```python
from build123d import *

# Parameters (mm, degrees)
BOSS_EXTRUDE1_DEPTH     = 40
SKETCH2_W               = 13.73333333
SKETCH2_H               = 6
CUT_EXTRUDE1_DEPTH      = 58.827329179
SKETCH3_W               = 40
SKETCH3_H               = 11.8
BOSS_EXTRUDE2_DEPTH     = 4
BOSS_EXTRUDE3_DEPTH     = 13.73333333
SKETCH10_R              = 1.47
BOSS_EXTRUDE7_DEPTH     = 5.5
SKETCH13_W              = 40
SKETCH13_H              = 44
BOSS_EXTRUDE8_DEPTH     = 19.5
CHAMFER2_START          = -20
CHAMFER2_DEPTH          = 5.5
EXTRUDE_THIN1_START     = -3
SKETCH14_R              = 9.05
SKETCH14_R_2            = 6.05
EXTRUDE_THIN1_DEPTH     = 8
BOSS_EXTRUDE9_START     = 3
BOSS_EXTRUDE9_DEPTH     = 3
FILLET1_START           = -31.5
FILLET1_DEPTH           = 11
SKETCH16_W              = 30
SKETCH16_H              = 18.101031733
CUT_EXTRUDE4_DEPTH      = 37.5
CHAMFER1_SIZE           = 14
CHAMFER1_SIZE2          = 18.1
SKETCH17_R              = 1.45
CUT_EXTRUDE5_DEPTH      = 35
SKETCH18_R              = 6.05
CUT_EXTRUDE6_DEPTH      = 16
FILLET2_R               = 0.6
CUT_EXTRUDE7_DEPTH      = 58.690987254
CUT_EXTRUDE7_DEPTH_BACK = 10


with BuildPart() as part:
    # Sketch1 → Boss-Extrude1 (new body)
    with BuildSketch(Plane.XY):
        Polygon((-20, -0.2), (-20, -12), (20, -12), (20, -0.2), (14.253501692, -0.2), (14.253501692, -1.22065898), (16.532842712, -3.5), (13.832842712, -6.2), (6.167157288, -6.2), (3.467157288, -3.5), (5.746498308, -1.22065898), (5.746498308, -0.2), (-5.746498308, -0.2), (-5.746498308, -1.22065898), (-3.467157288, -3.5), (-6.167157288, -6.2), (-13.832842712, -6.2), (-16.532842712, -3.5), (-14.253501692, -1.22065898), (-14.253501692, -0.2), align=None)
    extrude(amount=-BOSS_EXTRUDE1_DEPTH)

    # Sketch2 → Cut-Extrude1 (cut, through all)
    with BuildSketch(Plane.ZY.offset(20)):
        with Locations((-20, -3.2)):
            Rectangle(SKETCH2_W, SKETCH2_H)
    extrude(amount=-CUT_EXTRUDE1_DEPTH, mode=Mode.SUBTRACT)

    # Sketch3 → Boss-Extrude2 (add)
    with BuildSketch(Plane.XY):
        with Locations((0, -6.1)):
            Rectangle(SKETCH3_W, SKETCH3_H)
    extrude(amount=BOSS_EXTRUDE2_DEPTH)

    # Sketch4 → Boss-Extrude3 (add)
    with BuildSketch(Plane.XY.offset(-26.866666665)):
        Polygon((-20, -0.2), (-20, -6.2), (-13.832842712, -6.2), (-16.532842712, -3.5), align=None)
        Polygon((-6.167157288, -6.2), (6.167157288, -6.2), (3.467157288, -3.5), (0, -0.2), (-3.467157288, -3.5), align=None)
        Polygon((13.832842712, -6.2), (20, -6.2), (20, -0.2), (16.532842712, -3.5), align=None)
    extrude(amount=BOSS_EXTRUDE3_DEPTH)

    # Sketch10 → Boss-Extrude7 (add)
    with BuildSketch(Plane.ZY.offset(20)):
        with BuildLine():
            Line((-40, -12.8), (-42.5, -12.8))
            ThreePointArc((-42.5, -12.8), (-46.5, -8.8), (-42.5, -4.8))
            Line((-42.5, -4.8), (-40, -4.8))
            ThreePointArc((-40, -4.8), (-36, -8.8), (-40, -12.8))
        make_face()
        with Locations((-42.5, -8.8)):
            Circle(SKETCH10_R, mode=Mode.SUBTRACT)
    boss_extrude7 = extrude(amount=-BOSS_EXTRUDE7_DEPTH)

    # Sketch13 → Boss-Extrude8 (add)
    with BuildSketch(Plane.XZ.offset(12)):
        with Locations((0, -18)):
            Rectangle(SKETCH13_W, SKETCH13_H)
    extrude(amount=BOSS_EXTRUDE8_DEPTH)

    # Chamfer2: read off the stored shape, not the designer's step
    # Chamfer2 outline → Chamfer2 (add)
    with BuildSketch(Plane.YZ.offset(CHAMFER2_START)):
        with BuildLine():
            Line((-20.621590418, -40), (-12.177597262, -44.642857143))
            ThreePointArc((-12.177597262, -44.642857143), (-12.641249084, -43.615708508), (-12.8, -42.5))
            Line((-12.8, -42.5), (-12.8, -40))
            Line((-12.8, -40), (-20.621590418, -40))
        make_face()
    chamfer2 = extrude(amount=CHAMFER2_DEPTH)

    # Mirror1: Boss-Extrude7, Chamfer2 across plane
    add(boss_extrude7.mirror(Plane(origin=(0, 0, 0), x_dir=(0, 0, 1), z_dir=(1, 0, 0))))
    add(chamfer2.mirror(Plane(origin=(0, 0, 0), x_dir=(0, 0, 1), z_dir=(1, 0, 0))))

    # Sketch14 → Extrude-Thin1 (add)
    with BuildSketch(Plane.XZ.offset(31.5).offset(EXTRUDE_THIN1_START)):
        with Locations((-0.2, -42.5)):
            Circle(SKETCH14_R)
        with Locations((-0.2, -42.5)):
            Circle(SKETCH14_R_2, mode=Mode.SUBTRACT)
    extrude(amount=-EXTRUDE_THIN1_DEPTH)

    # Sketch15 → Boss-Extrude9 (add)
    with BuildSketch(Plane.XZ.offset(28.5).offset(BOSS_EXTRUDE9_START)):
        with BuildLine():
            Line((8.497844561, -40), (-8.897844561, -40))
            ThreePointArc((-8.897844561, -40), (-0.2, -51.55), (8.497844561, -40))
        make_face()
    extrude(amount=-BOSS_EXTRUDE9_DEPTH)

    # Fillet1: read off the stored shape, not the designer's step
    # Fillet1 outline → Fillet1 (add)
    with BuildSketch(Plane(origin=(0, 0, 0), x_dir=(1, 0, 0), z_dir=(0, 1, 0)).offset(FILLET1_START)):
        with BuildLine():
            ThreePointArc((20, 40), (12.845609752, 42.00741501), (7.532507128, 47.202215809))
            ThreePointArc((7.532507128, 47.202215809), (8.769787751, 43.7022511), (8.497844561, 40))
            Line((8.497844561, 40), (20, 40))
        make_face()
        with BuildLine():
            ThreePointArc((-8.897844561, 40), (-9.170229006, 43.698954374), (-7.935961427, 47.196530719))
            ThreePointArc((-7.935961427, 47.196530719), (-13.07347783, 42.098748758), (-20, 40))
            Line((-20, 40), (-8.897844561, 40))
        make_face()
    extrude(amount=FILLET1_DEPTH)

    # Sketch16 → Cut-Extrude4 (cut)
    with BuildSketch(Plane.XY.offset(4)):
        with Locations((0, -22.449484134)):
            Rectangle(SKETCH16_W, SKETCH16_H)
    extrude(amount=-CUT_EXTRUDE4_DEPTH, mode=Mode.SUBTRACT)

    # Chamfer1
    chamfer1_edges = [part.edges().sort_by_distance(p)[0] for p in [
        (0, -13.398968267, -33.5),
    ]]
    chamfer1_side = [part.faces().sort_by_distance(p)[0] for p in [
        (0, -13.398968267, -14.75),
    ]]
    chamfer(chamfer1_edges, length=CHAMFER1_SIZE, length2=CHAMFER1_SIZE2, reference=chamfer1_side[0])

    # Sketch17 → Cut-Extrude5 (cut)
    with BuildSketch(Plane.ZY.offset(20)):
        with Locations((-4, -26.5)):
            Circle(SKETCH17_R)
        with Locations((-25, -26.5)):
            Circle(SKETCH17_R)
    cut_extrude5 = extrude(amount=-CUT_EXTRUDE5_DEPTH, mode=Mode.SUBTRACT)

    # Mirror3: Cut-Extrude5 across plane
    add(cut_extrude5.mirror(Plane(origin=(0, 0, 0), x_dir=(0, 0, 1), z_dir=(1, 0, 0))), mode=Mode.SUBTRACT)

    # Sketch18 → Cut-Extrude6 (cut)
    with BuildSketch(Plane(origin=(0, -28.5, 0), x_dir=(1, 0, 0), z_dir=(0, 1, 0))):
        with Locations(Location((-0.2, 42.5, 0), (0, 0, 90))):
            Circle(SKETCH18_R)
    extrude(amount=CUT_EXTRUDE6_DEPTH, mode=Mode.SUBTRACT)

    # Fillet2
    fillet2_edges = [part.edges().sort_by_distance(p)[0] for p in [
        (16.695998577, -20.5, -40.066855447),
        (-16.826940077, -20.5, -40.066855447),
    ]]
    fillet(fillet2_edges, radius=FILLET2_R)

    # Sketch19 → Cut-Extrude7 (cut, two sides: drawn at the far end of the back side and taken through both)
    with BuildSketch(Plane(origin=(0, 0, -40), x_dir=(-1, 0, 0), z_dir=(0, 0, -1)).offset(-CUT_EXTRUDE7_DEPTH_BACK)):
        Polygon((16.532842712, -3.5), (15.232842712, -4.8), (14.5, -5.532842712), (13.832842712, -6.2), (10, -6.2), (10, -3.5), align=None)
        Polygon((-13.832842712, -6.2), (-14.5, -5.532842712), (-15.232842712, -4.8), (-16.532842712, -3.5), (-10, -3.5), (-10, -6.2), align=None)
    extrude(amount=CUT_EXTRUDE7_DEPTH + CUT_EXTRUDE7_DEPTH_BACK, mode=Mode.SUBTRACT)


solid = part.part
```
Geometry: final body of the model. Coordinates: model frame, mm. A direction names the side the tool comes from. Round coordinates to 2 decimals unless told otherwise and drop trailing zeros. Order: outer loops, then holes, each group sorted by start corner. A loop starts at its lowest first (then second) coordinate and runs counter-clockwise, first axis right, second up. Notation, with made-up numbers: (-3.75, 78) - (24.25, 78) arc R15 ccw to (24.25, 99) - close; hole circle Ø4 at (7.5, 41). An arc over 180 degrees is marked (long way). Write item = value, one per line. Start each with the question number.
Q1. Cut plane C-C on z = -10.5. Return the cut outline in (x, y), and give its area (3 significant figures).
Q2. Pin query (flat end, axial travel): pin 1 (3.5 mm diameter, centred on x = -16, y = -2, fed in from -Z); pin 2 (1 mm diameter, centred on x = -9, y = -23.5, fed in from +Z); pin 3 (3.5 mm diameter, centred on y = -8.8, z = -42.5, fed in from -X); pin 4 (1 mm diameter, centred on y = -22.5, z = -45.5, fed in from -X). Return the tip coordinate at first contact, or that it passes through.
Q3. Cut plane B-B on z = -4. Give the number of separate pieces and of enclosed holes in the cut face, and give its area (3 significant figures).
Q4. Pull-direction query (Y, two-part tool) for faces 5 (the flat face through (0, -9, 4)), 6 (the cylindrical face through (17.29, -7.75, -46.36)), 7 (the flat face through (4.591, -2.376, -33.341)), 8 (the flat face through (-17, -0.2, -33)); classes: +Y half, -Y half, draft (parallel to the pull), parting line (faces both ways), or undercut.
Q5. Cut plane D-D on y = -26.5. Return the cut outline in (x, z), and give its area (3 significant figures).
Q6. Cut plane A-A on y = -8.8. Return the cut outline in (x, z), and give its area (3 significant figures).
Q7. Ray query, line 1 (X direction, y = -14, z = -8.5); line 2 (Y direction, x = 18, z = -4); line 3 (X direction, y = -12, z = -43.5). Return the intervals inside material, ascending. Write a range as from..to.
Q8. Access query for faces 1 (the cylindrical face through (12.937, -25.639, -41.955)), 2 (the flat face through (-18, -2, -40)), 3 (the flat face through (-0.21, -22.58, -26.6)), 4 (the flat face through (4.591, -2.376, -6.475)). Directions: +Z, -Z, +X, -X, +Y, -Y. A direction counts if a zero-diameter tool reaches every point of the face in a straight line with its end or side. Return the directions, or none.
Outcome:
q1.outline = (-20, -31.5) - (-15, -31.5) - (-15, -13.4) - (15, -13.4) - (15, -31.5) - (20, -31.5) - (20, -0.2) - (14.25, -0.2) - (14.25, -1.22) - (16.53, -3.5) - (13.83, -6.2) - (6.17, -6.2) - (3.47, -3.5) - (5.75, -1.22) - (5.75, -0.2) - (-5.75, -0.2) - (-5.75, -1.22) - (-3.47, -3.5) - (-6.17, -6.2) - (-13.83, -6.2) - (-16.53, -3.5) - (-14.25, -1.22) - (-14.25, -0.2) - (-20, -0.2) - close
q1.area = 586 mm^2
q2.pin_1 = -40
q2.pin_2 = -26.93
q2.pin_3 = -20
q2.pin_4 = -9.56
q3.separate_pieces = 3
q3.enclosed_holes = 0
q3.area = 557 mm^2
q4.face_5 = draft
q4.face_6 = parting line
q4.face_7 = undercut
q4.face_8 = +Y half
q5.outline = (-20, -40) arc R15 cw to (-7.94, -47.2) arc R9.05 ccw to (7.53, -47.2) arc R15 cw to (20, -40) - (20, -26.45) - (15, -26.45) - (15, -29.63) - (-15, -29.63) - (-15, -26.45) - (-20, -26.45) - close; (-20, -23.55) - (-15, -23.55) - (-15, -5.45) - (-20, -5.45) - close; (-20, -2.55) - (-15, -2.55) - (-15, 4) - (-20, 4) - close; (15, -23.55) - (20, -23.55) - (20, -5.45) - (15, -5.45) - close; (15, -2.55) - (20, -2.55) - (20, 4) - (15, 4) - close; hole circle Ø12.1 at (-0.2, -42.5)
q5.area = 791 mm^2
q6.outline = (-20, -46.5) - (-14.5, -46.5) - (-14.5, -43.97) - (-20, -43.97) - close; (-20, -41.03) - (-14.5, -41.03) - (-14.5, -40) - (14.5, -40) - (14.5, -41.03) - (20, -41.03) - (20, 4) - (-20, 4) - close; (14.5, -46.5) - (20, -46.5) - (20, -43.97) - (14.5, -43.97) - close
q6.area = 1,800 mm^2
q7.line_1 = -20..-15, 15..20
q7.line_2 = -31.5..-27.95, -25.05..-0.2
q7.line_3 = -20..-14.5, 14.5..20
q8.face_1 = -Z, +X, -Y
q8.face_2 = -Z, +X, -X, +Y
q8.face_3 = +Z, -Y
q8.face_4 = -Z
